Read the model definition and answer for the solid it produces. Units are mm, in the model's axes. Face numbers are marked on the shaded views. A direction names the side the tool comes from. Coordinates: 2 decimals unless noted, no trailing zeros. Order: outer loops, then holes, each group sorted by start corner. A loop starts at its lowest first (then second) coordinate and runs counter-clockwise, first axis right, second up. Notation, with made-up numbers: (41.5, 89.25) -> (47.5, 89.25) arc R4 cw to (47.5, 93.25) -> close; hole circle Ø6 at (63.5, 18.5). An arc over 180 degrees is marked (long way). Answer as a JSON object with one key per item and string values. Group by question number.
1) Determine the mould class of the marked faces 1, 2 and 3 for opening direction X: released by +X, released by -X, zero draft, split by the parting line, or undercut.
2) Section D-D on z = 20 is taken. Determine the outline of the cut face in (x, y), and give its area (3 significant figures).
3) Consider L1, parallel to Y at x = 0, z = 18.75; L2, parallel to Z at x = -52.5, y = 40.5; L3, parallel to X at y = -10, z = 19.5. Determine where each line is inside the solid, lowest interval first.
4) A tool of negligible diameter and unlimited length cuts with its end or side. For the marked faces 4, 5 and 6, from which of +Z, -Z, +X, -X, +Y, -Y can it reach the whole face along a straight path? Write none if from no direction.
5) Given pin 1 (9.5 mm diameter, centred on y = -22.5, z = -11.5, fed in from -X); pin 2 (1.5 mm diameter, centred on x = -61.5, z = 1, fed in from +Y); pin 3 (14.5 mm diameter, centred on x = 12, y = 6, fed in from +Z), each flat-ended and moving along its own axis, determine where each tip first touches the part or whether it passes through.
6) Section A-A on x = 0 is taken. Determine the outline of the cut face in (y, z).
7) Section C-C on y = 0 is taken. Determine the outline of the cut face in (x, z), and give its area (3 significant figures).
8) Section B-B on z = -15 is taken. Determine the outline of the cut face in (x, y).
from build123d import *

# Parameters (mm, degrees)
SKETCH1_R           = 90.043
BOSS_EXTRUDE1_DEPTH = 10
SKETCH3_W           = 40
SKETCH3_H           = 10
BOSS_EXTRUDE2_DEPTH = 40
BOSS_EXTRUDE5_DEPTH = 5
SKETCH5_R           = 28.5
SKETCH5_R_2         = 24.5
BOSS_EXTRUDE6_DEPTH = 15
SKETCH6_R           = 24.5
SKETCH6_R_2         = 16.821657313
BOSS_EXTRUDE7_DEPTH = 3


with BuildPart() as part:
    # Sketch1 → Boss-Extrude1 (new body)
    with BuildSketch(Plane.XY):
        Circle(SKETCH1_R)
    extrude(amount=BOSS_EXTRUDE1_DEPTH)

    # Sketch3 → Boss-Extrude2 (add)
    with BuildSketch(Plane(origin=(0, 0, 0), x_dir=(-1, 0, 0), z_dir=(0, 0, -1))):
        with Locations((0, -40)):
            Rectangle(SKETCH3_W, SKETCH3_H)
    extrude(amount=BOSS_EXTRUDE2_DEPTH)

    # Sketch4 → Boss-Extrude5 (add)
    with BuildSketch(Plane.ZY.offset(20)):
        Polygon((-40, -35), (0, -15.575750454), (0, -20.206895082), (-30.463169004, -35), align=None)
    boss_extrude5 = extrude(amount=-BOSS_EXTRUDE5_DEPTH)

    # Mirror1: Boss-Extrude5 across plane
    add(boss_extrude5.mirror(Plane(origin=(0, 0, 0), x_dir=(0, 0, 1), z_dir=(1, 0, 0))))

    # Sketch5 → Boss-Extrude6 (add)
    with BuildSketch(Plane.XY.offset(10)):
        Circle(SKETCH5_R)
        Circle(SKETCH5_R_2, mode=Mode.SUBTRACT)
    extrude(amount=BOSS_EXTRUDE6_DEPTH)

    # Sketch6 → Boss-Extrude7 (add)
    with BuildSketch(Plane.XY.offset(10)):
        Circle(SKETCH6_R)
        Circle(SKETCH6_R_2, mode=Mode.SUBTRACT)
    extrude(amount=BOSS_EXTRUDE7_DEPTH)


solid = part.part
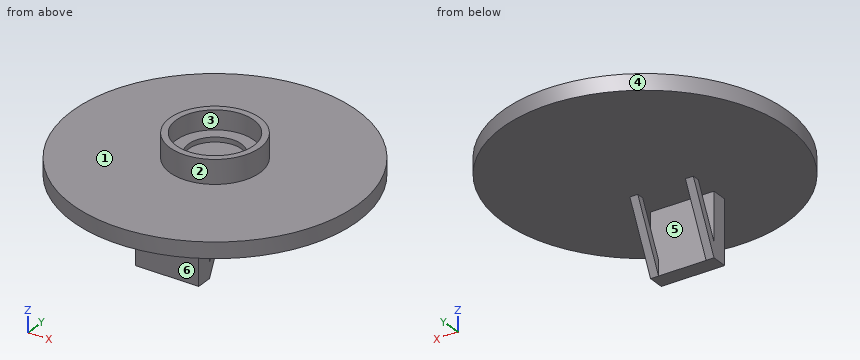
Worked answers:
{
 "1": {"face 1": "zero draft", "face 2": "split by the parting line", "face 3": "undercut"},
 "2": {"outline": "circle Ø57 at (0, 0); hole circle Ø49 at (0, 0)", "area": "666 mm²"},
 "3": {"L1": "y = -28.5 to -24.5, 24.5 to 28.5", "L2": "z = 0 to 10", "L3": "x = -26.69 to -22.37, 22.37 to 26.69"},
 "4": {"face 4": "+Z, -Z", "face 5": "none", "face 6": "-Z, +X, -X, -Y"},
 "5": {"pin 1": "stops at x = -20", "pin 2": "stops at y = 66.46", "pin 3": "stops at z = 13"},
 "6": {"outline": "(-90.04, 0) -> (-45, 0) -> (-45, -40) -> (-35, -40) -> (-35, 0) -> (90.04, 0) -> (90.04, 10) -> (28.5, 10) -> (28.5, 25) -> (24.5, 25) -> (24.5, 13) -> (16.82, 13) -> (16.82, 10) -> (-16.82, 10) -> (-16.82, 13) -> (-24.5, 13) -> (-24.5, 25) -> (-28.5, 25) -> (-28.5, 10) -> (-90.04, 10) -> close"},
 "7": {"outline": "(-90.04, 0) -> (90.04, 0) -> (90.04, 10) -> (28.5, 10) -> (28.5, 25) -> (24.5, 25) -> (24.5, 13) -> (16.82, 13) -> (16.82, 10) -> (-16.82, 10) -> (-16.82, 13) -> (-24.5, 13) -> (-24.5, 25) -> (-28.5, 25) -> (-28.5, 10) -> (-90.04, 10) -> close", "area": "1,970 mm²"},
 "8": {"outline": "(-20, -45) -> (20, -45) -> (20, -35) -> (-20, -35) -> close; (-20, -27.49) -> (-15, -27.49) -> (-15, -22.86) -> (-20, -22.86) -> close; (15, -27.49) -> (20, -27.49) -> (20, -22.86) -> (15, -22.86) -> close"}
}
